Can you work these out from the model? Positions are in its coordinate system, mm. Face numbers are marked on the shaded views. Round coordinates to 2 decimals unless told otherwise and drop trailing zeros. Loops run counter-clockwise (first coordinate to the right, second up) from the corner with the lowest first, then second, coordinate; pieces in that order, holes last.
(1) Will these pins go through, and if not, where does the flat tip stop? pin 1 Ø1.4 at (x, y) = (-0.5, 0.5) entering from -Z; pin 2 Ø1 at (y, z) = (37, 15.5) entering from +X; pin 3 Ø4 at (y, z) = (62, 16.5) entering from +X; pin 4 Ø1 at (x, y) = (-1.5, 34.5) entering from +Z.
(2) I want a section at D-D on y = 62. Write out the boundary of the cut face in (x, z).
(3) I want a section at A-A on z = 3. Write out the boundary of the cut face in (x, y), plus the area to 3 significant figures.
(4) I want a section at C-C on z = -10. Write out the boundary of the cut face in (x, y).
(5) If I drill on line 1 along Y through (x, z) = (0.1, -4); line 2 along Y through (x, z) = (0.7, 6); line 3 along Z through (x, y) = (0.1, 39.5), over which ranges is the centre line in solid material (lowest first)?
(6) Thinking about a two-plate mould opening in Y: for the marked faces 1 and 2, which applies, released by +Y, released by -Y, zero draft, split by the parting line, or undercut?
(7) I want a section at B-B on x = 0. Write out the boundary of the cut face in (y, z), plus the area to 3 significant figures.
from build123d import *

# Parameters (mm, degrees)
F1_R = 2.38125


with BuildPart() as f2:
    # F2: sweep along a path in F0
    with BuildLine(Plane.YZ) as f2_path:
        Line((0, 0), (0, 12.7))
        ThreePointArc((0, 12.7), (1.3949039546, 16.0675960454), (4.7625, 17.4625))
        Line((4.7625, 17.4625), (96.8375, 17.4625))
        ThreePointArc((96.8375, 17.4625), (100.2050960454, 16.0675960454), (101.6, 12.7))
        Line((101.6, 12.7), (101.6, -6.35))
    # F1 (on Top) → F2 (sweep)
    with BuildSketch(Plane.XY):
        Circle(F1_R)
    sweep(path=f2_path.line)

    # F0 (on Right) → F3 (revolve)
    with BuildSketch(Plane.YZ):
        with BuildLine():
            Line((103.98125, -6.35), (101.6, -6.35))
            Line((101.6, -6.35), (101.6, -13.5071065476))
            Line((101.6, -13.5071065476), (101.6, -14.2875))
            ThreePointArc((101.6, -14.2875), (102.088655971, -14.1155712405), (102.362, -13.6755403345))
            Line((102.362, -13.6755403345), (103.98125, -6.35))
        make_face()
    revolve(axis=Axis((0, 101.6, -9.9285532738), (0, 0, -1)))


solid = f2.part
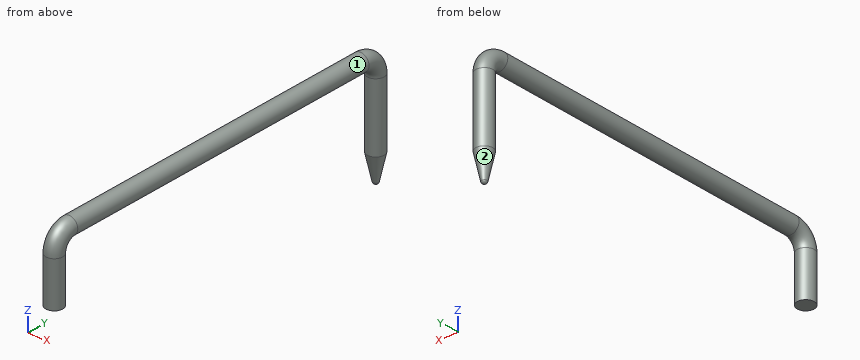
Filled sheet:
1. pin 1: stops at z = 0
1. pin 2: stops at x = 1.88
1. pin 3: stops at x = 2.38
1. pin 4: stops at z = 19.62
2. outline: circle Ø4.76 at (0, 17.46)
3. outline: circle Ø4.76 at (0, 0); circle Ø4.76 at (0, 101.6)
3. area: 35.6 mm2
4. outline: circle Ø3.15 at (0, 101.6)
5. line 1: y = 99.22 to 103.98
5. line 2: y = -2.28 to 2.28, 99.32 to 103.88
5. line 3: z = 15.08 to 19.84
6. face 1: undercut
6. face 2: split by the parting line
7. outline: (-2.38, 0) - (2.38, 0) - (2.38, 12.7) arc R2.38 cw to (4.76, 15.08) - (96.84, 15.08) arc R2.38 cw to (99.22, 12.7) - (99.22, -6.35) - (100.84, -13.68) arc R0.78 ccw to (102.36, -13.68) - (103.98, -6.35) - (103.98, 12.7) arc R7.14 ccw to (96.84, 19.84) - (4.76, 19.84) arc R7.14 ccw to (-2.38, 12.7) - close
7. area: 685 mm2
